from build123d import *

# Parameters (mm, degrees)
F1_DEPTH = 5.08


# Not quite as in the source:
# - a feature names something its author has since deleted; it is built from what else it names


with BuildPart() as f1:
    # F0 (on Top) → F1 (new body)
    with BuildSketch(Plane.XY):
        Polygon((-43.18, 9.525), (-43.18, 0), (0, 0), (0, 19.05), (-19.05, 19.05), (-19.05, 13.97), (-24.13, 13.97), (-24.13, 19.05), (-38.1, 19.05), (-43.18, 19.05), (-43.18, 14.605), (-38.1, 14.605), (-38.1, 9.525), align=None)
        Polygon((-43.18, -14.605), (-43.18, -19.05), (-24.13, -19.05), (-24.13, -13.97), (-19.05, -13.97), (-19.05, -19.05), (19.05, -19.05), (19.05, -13.97), (24.13, -13.97), (24.13, -19.05), (43.18, -19.05), (43.18, -14.605), (38.1, -14.605), (38.1, -9.525), (43.18, -9.525), (43.18, 0), (0, 0), (-43.18, 0), (-43.18, -9.525), (-38.1, -9.525), (-38.1, -14.605), align=None)
        Polygon((0, 19.05), (0, 0), (43.18, 0), (43.18, 9.525), (38.1, 9.525), (38.1, 14.605), (43.18, 14.605), (43.18, 19.05), (38.1, 19.05), (24.13, 19.05), (24.13, 13.97), (19.05, 13.97), (19.05, 19.05), align=None)
    extrude(amount=F1_DEPTH)


solid = f1.part
Can you work these out from the model? Positions are in its coordinate system, mm. A direction names the side the tool comes from. Round coordinates to 2 decimals unless told otherwise and drop trailing zeros. Order: outer loops, then holes, each group sorted by start corner. A loop starts at its lowest first (then second) coordinate and runs counter-clockwise, first axis right, second up. Notation, with made-up numbers: (21.5, 35) - (26.5, 35) arc R18 ccw to (26.5, 54) - close; hole circle Ø7 at (15, 44.25). An arc over 180 degrees is marked (long way). Answer in a Markdown table with one row per item.
(1) If we mould it in two halves opening along X, with no side actions, what happens to faces 1 (the face through (-43.18, 0, 3)), 2 (the face through (-22, 13.97, 3)), 3 (the face through (-1, 0, 5.08))? For each: released by +X, released by -X, zero draft, split by the parting line, or undercut.
From the geometry:
| item | result |
|---|---|
| face 1 | released by -X |
| face 2 | undercut |
| face 3 | zero draft |
(2) For P1, Ø2, axis at x = 20.5, z = 2, coming from the +Y side; P2, Ø1.5, axis at y = 11, z = 0.5, coming from the -X side; P3, Ø1, axis at y = -12, z = 4, coming from the +X side, each with a flat end and sliding along its axis, tell me the tip position at first contact or that it passes through.
From the geometry:
| item | result |
|---|---|
| P1 | stops at y = 13.97 |
| P2 | stops at x = -38.1 |
| P3 | stops at x = 38.1 |
(3) Suppose I cut it at A-A, the plane y = 11. Please give me the cut outline in (x, z), plus the area to 3 significant figures.
From the geometry:
| item | result |
|---|---|
| outline | (-38.1, 0) - (38.1, 0) - (38.1, 5.08) - (-38.1, 5.08) - close |
| area | 387 mm2 |
(4) Please list where these lines run through material, in increasing order: L1, parallel to X at y = -15, z = 1.05; L2, parallel to X at y = -12, z = 2.6; L3, parallel to Y at x = -21.5, z = 3.1. Write a range as from..to.
From the geometry:
| item | result |
|---|---|
| L1 | x = -43.18..-24.13, -19.05..19.05, 24.13..43.18 |
| L2 | x = -38.1..38.1 |
| L3 | y = -13.97..13.97 |
(5) Which directions (+Z, -Z, +X, -X, +Y, -Y) give clear straight access to the entire face, cutting with the end or side of a thin tool? Please do faces 4 (the face through (-22, -13.97, 3)), 5 (the face through (-41, 14.605, 3)), 6 (the face through (41, 14.605, 3)), 7 (the face through (-24.13, 16, 3)).
From the geometry:
| item | result |
|---|---|
| face 4 | +Z, -Z, -Y |
| face 5 | +Z, -Z, -X |
| face 6 | +Z, -Z, +X |
| face 7 | +Z, -Z, +Y |
